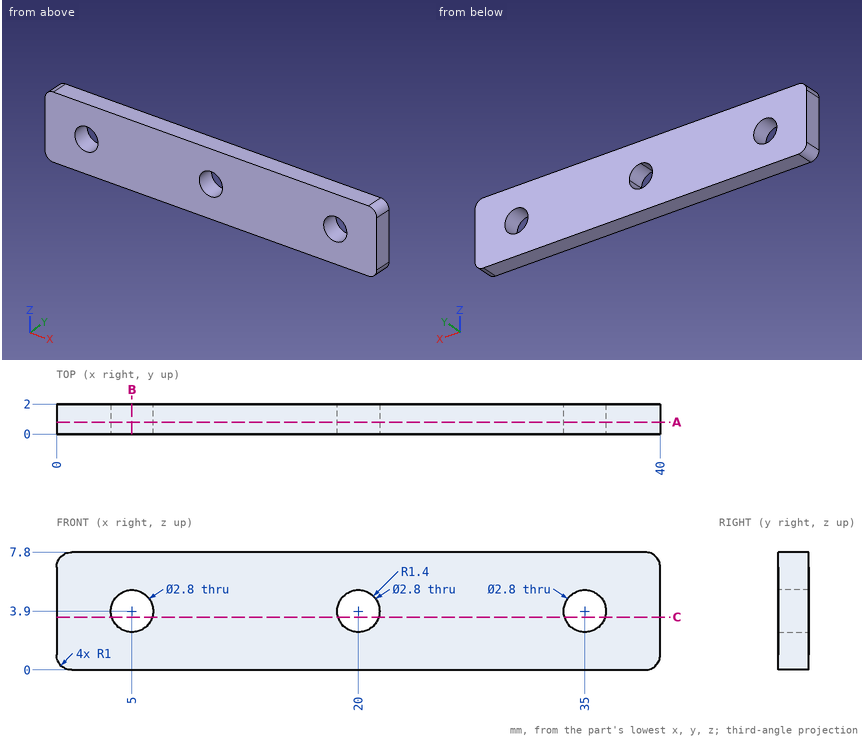
Verification items for this drawing (mm, ordinates from the low corner). Round coordinates to 2 decimals unless told otherwise and drop trailing zeros. Loops run counter-clockwise (first coordinate to the right, second up) from the corner with the lowest first, then second, coordinate; pieces in that order, holes last. Notation, with made-up numbers: (56.25, 37) - (68.25, 37) arc R13 ccw to (68.25, 61) - close; hole circle Ø11 at (-30.75, -22). An arc over 180 degrees is marked (long way). Answer as CSV lines item,"result". Start each with the question number.
Item 1: Section check B-B (x = 5). Record the boundary of the cut face in (y, z), and give its area (4 significant figures).
Item 2: Scan lines: line 1 (X direction, y = 0.6, z = 4); line 2 (Z direction, x = 5, y = 1.1); line 3 (X direction, y = 1.25, z = 3.5). Record each from-to range of solid material in increasing order. Write a range as [from, to].
Item 3: Section check A-A (y = 0.8). Record the boundary of the cut face in (x, z).
Item 4: Section check C-C (z = 3.5). Record the boundary of the cut face in (x, y), and give its area (3 significant figures).
Report:
1,outline,"(0, 0) - (2, 0) - (2, 2.5) - (0, 2.5) - close; (0, 5.3) - (2, 5.3) - (2, 7.8) - (0, 7.8) - close"
1,area,"10.00 mm2"
2,line 1,"x = [0, 3.6], [6.4, 18.6], [21.4, 33.6], [36.4, 40]"
2,line 2,"z = [0, 2.5], [5.3, 7.8]"
2,line 3,"x = [0, 3.66], [6.34, 18.66], [21.34, 33.66], [36.34, 40]"
3,outline,"(0, 1) arc R1 ccw to (1, 0) - (39, 0) arc R1 ccw to (40, 1) - (40, 6.8) arc R1 ccw to (39, 7.8) - (1, 7.8) arc R1 ccw to (0, 6.8) - close; hole circle Ø2.8 at (5, 3.9); hole (20, 5.3) arc R1.4 ccw (long way) to (21.4, 3.9) arc R1.4 ccw to start; hole circle Ø2.8 at (35, 3.9)"
4,outline,"(0, 0) - (3.66, 0) - (3.66, 2) - (0, 2) - close; (6.34, 0) - (18.66, 0) - (18.66, 2) - (6.34, 2) - close; (21.34, 0) - (33.66, 0) - (33.66, 2) - (21.34, 2) - close; (36.34, 0) - (40, 0) - (40, 2) - (36.34, 2) - close"
4,area,"63.9 mm2"
